Build history of the part. All positions in model axes, mm. A direction names the side the tool comes from. Round coordinates to 2 decimals unless told otherwise and drop trailing zeros. Write each loop counter-clockwise with the first axis right and the second up, starting at its lowest first coordinate (ties: lowest second). Pieces come first, ordered by that corner, then holes. Notation, with made-up numbers: M -25.75,-30 L 1.25,-30 A13 ccw 1.25,-16 Z; hole C -39.75,-30.75 d4. An arc over 180 degrees is marked long. Use a Markdown table: item, result.
from build123d import *

# Parameters (mm, degrees)
F1_DEPTH = 75
F2_W     = 30
F2_H     = 40
F2_R     = 2.65
F3_DEPTH = 5
F4_W     = 4.85
F4_H     = 40
F5_DEPTH = 20
F6_R     = 2.65
F7_DEPTH = 30
F9_DEPTH = 30


with BuildPart() as f1:
    # F0 (on Top) → F1 (new body)
    with BuildSketch(Plane.XY):
        with BuildLine():
            Line((15, 0), (-15, 0))
            ThreePointArc((-15, 0), (0, -15), (15, 0))
        make_face()
    extrude(amount=F1_DEPTH)

    # F2 (on Top) → F3 (join)
    with BuildSketch(Plane.XY):
        with Locations((0, -20)):
            Rectangle(F2_W, F2_H)
        with Locations((0, -30)):
            Circle(F2_R, mode=Mode.SUBTRACT)
    extrude(amount=F3_DEPTH)

    # F4 (on face) → F5 (join)
    with BuildSketch(Plane(origin=(0, 0, 0), x_dir=(1, 0, 0), z_dir=(0, 0, -1))):
        with Locations((-12.575, 20)):
            Rectangle(F4_W, F4_H)
        with Locations((12.575, 20)):
            Rectangle(F4_W, F4_H)
    extrude(amount=F5_DEPTH)

    # F6 (on face) → F7 (cut, through all)
    with BuildSketch(Plane(origin=(-15, 0, 0), x_dir=(0, -1, 0), z_dir=(-1, 0, 0))):
        with Locations((30, -10)):
            Circle(F6_R)
    extrude(amount=-F7_DEPTH, mode=Mode.SUBTRACT)

    # F8 (on face) → F9 (cut, through all)
    with BuildSketch(Plane.YZ.offset(15)):
        Polygon((0, 0), (-20, -20), (0, -20), align=None)
    extrude(amount=-F9_DEPTH, mode=Mode.SUBTRACT)


solid = f1.part
Q1. Two-plate mould, pull along Z, no slides. Class faces 1 (the flat face through (15, -25, -5)), 2 (the cylindrical face through (-12.609, -27.353, -9.883)), 3 (the flat face through (0, -6, 75)): +Z half, -Z half, draft (parallel to the pull), parting line (faces both ways), or undercut.
Response values:
| item | result |
|---|---|
| face 1 | draft |
| face 2 | undercut |
| face 3 | +Z half |
Q2. Cut at A-A on x = 0. Give the cut face in (y, z), and give its area (3 significant figures).
Response values:
| item | result |
|---|---|
| outline | M -40,0 L -32.65,0 L -32.65,5 L -40,5 Z; M -27.35,0 L 0,0 L 0,75 L -15,75 L -15,5 L -27.35,5 Z |
| area | 1,220 mm2 |
Q3. Cut at C-C on y = -30. Give the cut face in (x, z), and give its area (3 significant figures).
Response values:
| item | result |
|---|---|
| outline | M -15,-20 L -10.15,-20 L -10.15,-12.65 L -15,-12.65 Z; M -15,-7.35 L -10.15,-7.35 L -10.15,0 L -2.65,0 L -2.65,5 L -15,5 Z; M 2.65,0 L 10.15,0 L 10.15,-7.35 L 15,-7.35 L 15,5 L 2.65,5 Z; M 10.15,-20 L 15,-20 L 15,-12.65 L 10.15,-12.65 Z |
| area | 266 mm2 |
Q4. Cut at D-D on y = -25.5. Give the cut face in (x, z).
Response values:
| item | result |
|---|---|
| outline | M -15,-20 L -10.15,-20 L -10.15,0 L 10.15,0 L 10.15,-20 L 15,-20 L 15,5 L -15,5 Z |
Q5. Drill centre lines: L1, parallel to Z at x = -13.9, y = -30; L2, parallel to Z at x = -5, y = -12; L3, parallel to Z at x = -6, y = -28.5. Where is each one in solid material? Low to high.
Response values:
| item | result |
|---|---|
| L1 | z = -20 to -12.65, -7.35 to 5 |
| L2 | z = 0 to 75 |
| L3 | z = 0 to 5 |
Q6. Cut at B-B on z = -10. Give the cut face in (x, y).
Response values:
| item | result |
|---|---|
| outline | M -15,-40 L -10.15,-40 L -10.15,-32.65 L -15,-32.65 Z; M -15,-27.35 L -10.15,-27.35 L -10.15,-10 L -15,-10 Z; M 10.15,-40 L 15,-40 L 15,-32.65 L 10.15,-32.65 Z; M 10.15,-27.35 L 15,-27.35 L 15,-10 L 10.15,-10 Z |
Q7. Drop flat-ended pins along their axis: P1, Ø3, axis at y = -30, z = -10, coming from the -X side; P2, Ø6, axis at x = 0, z = 30, coming from the -Y side; P3, Ø5, axis at y = -9, z = 45.5, coming from the -X side. Give the stop position or say it passes through.
Response values:
| item | result |
|---|---|
| P1 | passes through |
| P2 | stops at y = -15 |
| P3 | stops at x = -13.52 |
Q8. Which spindle directions (+Z, -Z, +X, -X, +Y, -Y) get a long thin tool onto all of the face, cutting with end or side? Do faces 4 (the flat face through (0, -20, 0)), 5 (the cylindrical face through (0, -15, 40)), 6 (the flat face through (-4, -40, 1)). Say none if no direction does.
Response values:
| item | result |
|---|---|
| face 4 | -Z, +Y, -Y |
| face 5 | +Z, -Y |
| face 6 | +Z, -Z, +X, -X, -Y |
